Design review of the part shown in the three views and the two pictorial views. Dimensions are in mm from the part's minimum x, y and z. Give positions to 0.01 mm unless a question says otherwise; leave off trailing zeros. Order: outer loops, then holes, each group sorted by start corner. A loop starts at its lowest first (then second) coordinate and runs counter-clockwise, first axis right, second up.
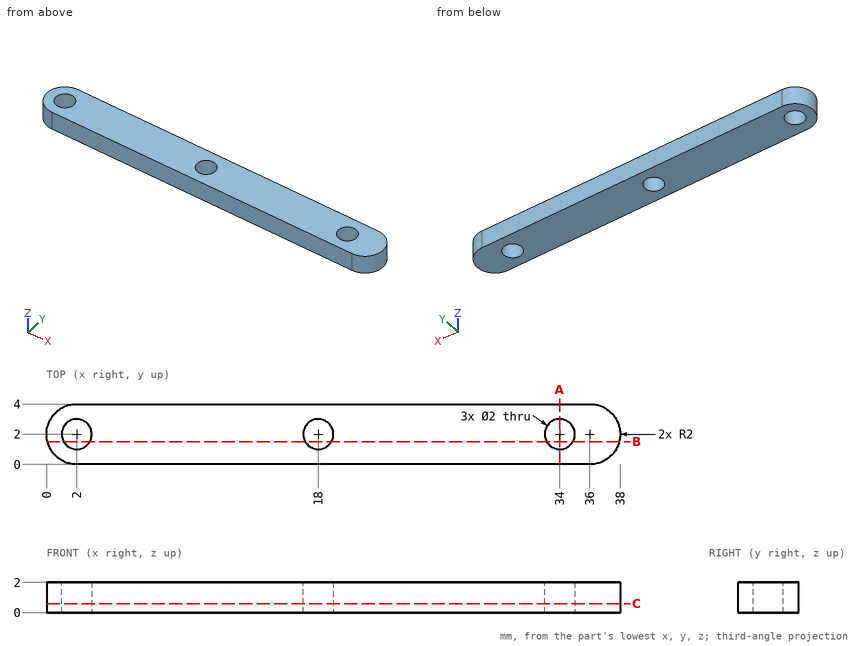
1) We need section B-B on y = 1.5. Give the boundary of the cut face in (x, z).
Answer sheet:
outline: (0.06, 0) - (1.13, 0) - (1.13, 2) - (0.06, 2) - close; (2.87, 0) - (17.13, 0) - (17.13, 2) - (2.87, 2) - close; (18.87, 0) - (33.13, 0) - (33.13, 2) - (18.87, 2) - close; (34.87, 0) - (37.94, 0) - (37.94, 2) - (34.87, 2) - close
2) We need section A-A on x = 34. Give the boundary of the cut face in (y, z).
Answer sheet:
outline: (0, 0) - (1, 0) - (1, 2) - (0, 2) - close; (3, 0) - (4, 0) - (4, 2) - (3, 2) - close
3) We need section C-C on z = 0.6. Give the boundary of the cut face in (x, y), then the cut area to 3 significant figures.
Answer sheet:
outline: (2, 0) - (36, 0) arc R2 ccw to (36, 4) - (2, 4) arc R2 ccw to start; hole circle Ø2 at (2, 2); hole circle Ø2 at (18, 2); hole circle Ø2 at (34, 2)
area: 139 mm2
4) To check wall thickness, follow line 1 (Y direction, x = 2, z = 1.25); line 2 (X direction, y = 1.3, z = 0.2); line 3 (X direction, y = 1.85, z = 0.75). State the ranges of each line that lie inside material, in increasing order.
Answer sheet:
line 1: y = 0 to 1, 3 to 4
line 2: x = 0.13 to 1.29, 2.71 to 17.29, 18.71 to 33.29, 34.71 to 37.87
line 3: x = 0.01 to 1.01, 2.99 to 17.01, 18.99 to 33.01, 34.99 to 37.99
